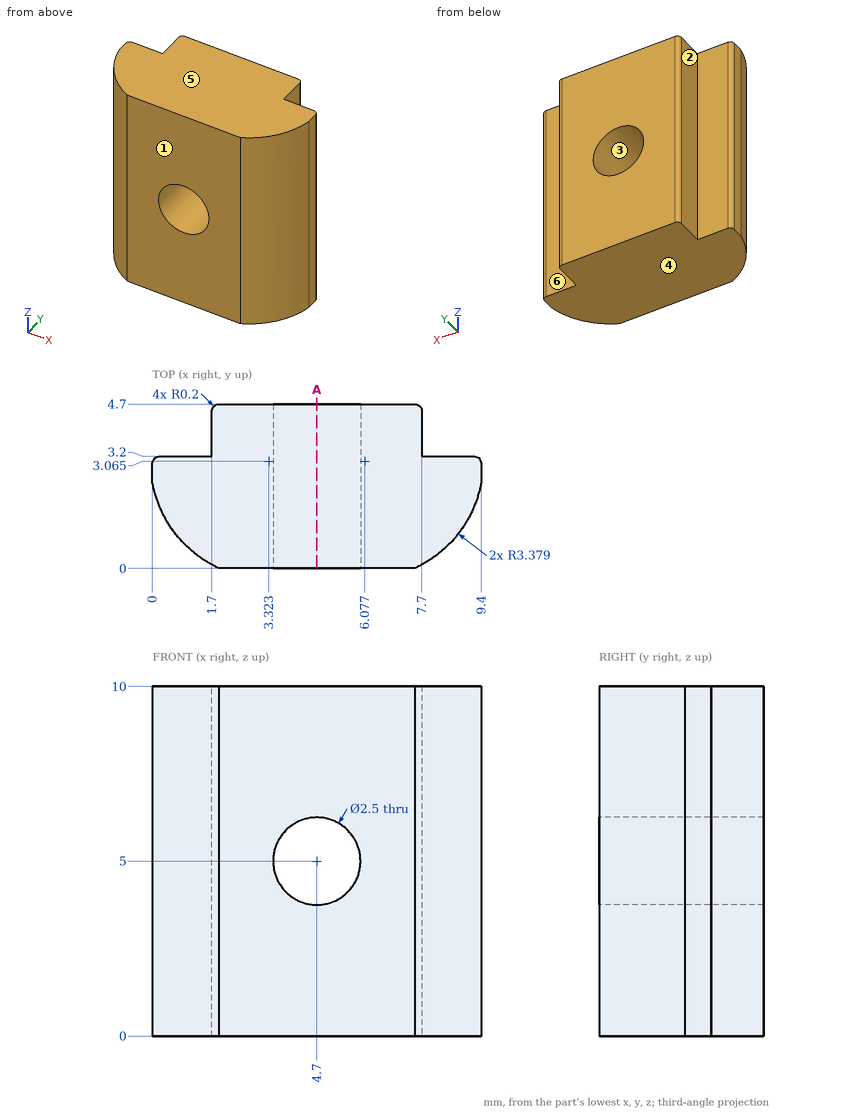
Job drawing, mm, ordinate dimensions from the low corner. One solid piece. A direction names the side the tool comes from. Give positions to 0.01 mm unless a question says otherwise; leave off trailing zeros. Order: outer loops, then holes, each group sorted by start corner. A loop starts at its lowest first (then second) coordinate and runs counter-clockwise, first axis right, second up. Notation, with made-up numbers: M 52,24.25 L 71,24.25 A16 ccw 71,35.25 Z; hole C 15,65 d2. An arc over 180 degrees is marked long. Return JSON: item names as keys, results as strings.
Q1. Flat gauge pins, fed straight in: pin 1 (0.6 mm diameter, centred on y = 4, z = 2.5, fed in from +X); pin 2 (1.6 mm diameter, centred on x = 9, z = 3, fed in from +Y). Where does each tip first touch, or does it go through?
Answer list:
{"pin 1": "stops at x = 7.7", "pin 2": "stops at y = 3.2"}
Q2. 3-axis set-ups, long thin cutter, end or side, ignore diameter. For the marked faces 1 and 2: which of +Z, -Z, +X, -X, +Y, -Y reach the whole face in a straight line?
Answer list:
{"face 1": "+Z, -Z, +X, -X, -Y", "face 2": "+Z, -Z, -X, +Y"}
Q3. Band-saw the part on A-A (x = 4.7). Give the cut face in (y, z).
Answer list:
{"outline": "M 0,0 L 4.7,0 L 4.7,3.75 L 0,3.75 Z; M 0,6.25 L 4.7,6.25 L 4.7,10 L 0,10 Z"}
Q4. Two-plate mould, pull along Z, no slides. Class the marked faces 3, 4, 5 and 6: pulls with the +Z half, pulls with the -Z half, needs draft (parallel to the pull), parting line crosses it, or undercut.
Answer list:
{"face 3": "undercut", "face 4": "pulls with the -Z half", "face 5": "pulls with the +Z half", "face 6": "needs draft"}
Q5. Wall check: probe 1 along X at (y, z) = (3.4, 5); probe 2 along Z at (x, y) = (5, 3.1); probe 3 along X at (y, z) = (4.05, 2.5). Give the ranges that are in metal, low to high. Write a range as from..to.
Answer list:
{"probe 1": "x = 1.7..3.45, 5.95..7.7", "probe 2": "z = 0..3.79, 6.21..10", "probe 3": "x = 1.7..7.7"}
